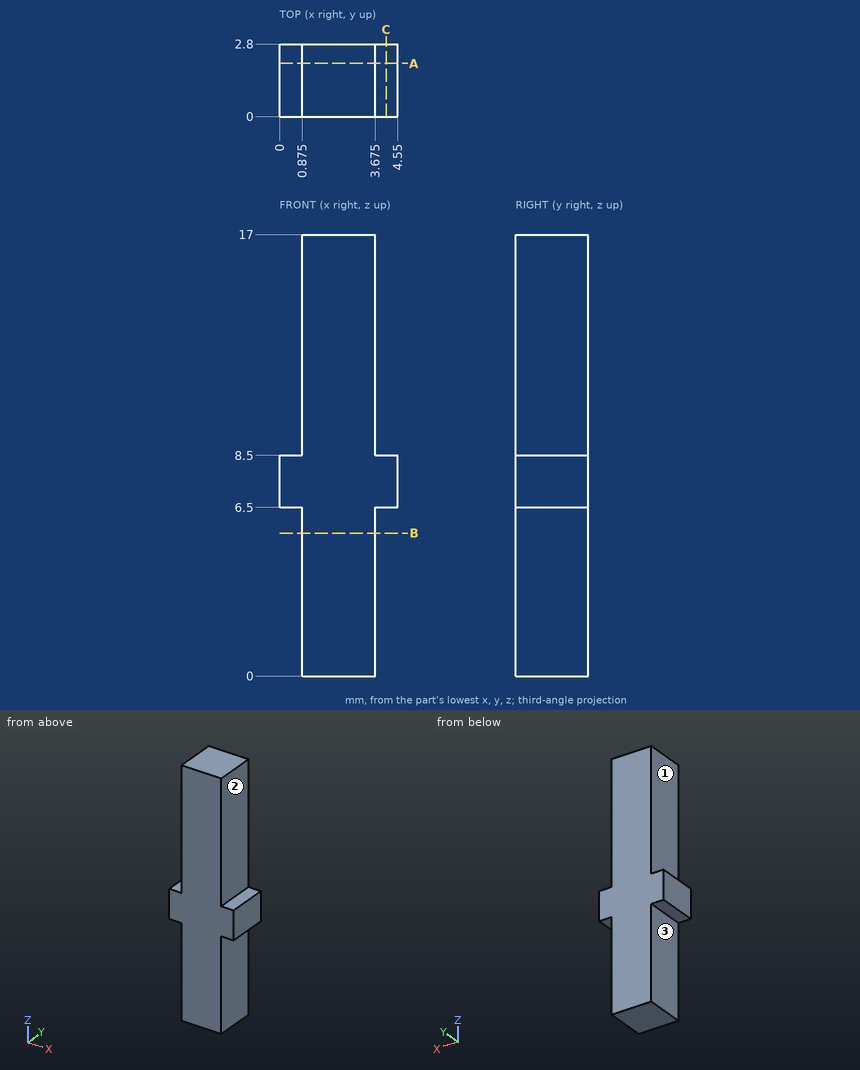
Study the drawing (mm; zero at the part's minimum x, y, z) and answer. A direction names the side the tool comes from. Give positions to 0.01 mm unless a question says otherwise; leave off trailing zeros. Order: outer loops, then holes, each group sorted by start corner. A loop starts at its lowest first (then second) coordinate and runs counter-clockwise, first axis right, second up. Notation, with made-up numbers: (63, 69.5) - (104, 69.5) arc R30 cw to (104, 92.5) - close; hole circle Ø6 at (71.5, 80). An arc over 180 degrees is marked (long way). Use one line per item in the form item = value. Start each with the question number.
(1) A cutting plane is placed at C-C, the plane x = 4.1. Write down the section's boundary in (y, z).
(2) A cutting plane is placed at B-B, the plane z = 5.5. Write down the section's boundary in (x, y) (3 decimals).
(3) A cutting plane is placed at A-A, the plane y = 2.05. Write down the section's boundary in (x, z) (3 decimals).
(4) Flat-ended cylindrical pins translate along their axes: pin 1 Ø0.8 at (y, z) = (1.5, 12) entering from +X (3 decimals); pin 2 Ø1.4 at (y, z) = (1.5, 11.5) entering from -X (3 decimals); pin 3 Ø1 at (x, y) = (4, 1) entering from -Z. Find the tip coordinate at first contact, or state that the pin passes through.
(5) Consider line 1 (X direction, y = 2.5, z = 5.25) (3 decimals); line 2 (Z direction, x = 0.7, y = 1.5). Determine where each line is inside the solid, lowest interval first. Write a range as from..to.
(6) For the marked faces 1, 2 and 3, determine the directions among +Z, -Z, +X, -X, +Y, -Y from which every point of the face is accessible in a straight line to the end or side of a thin tool.
Ans:
q1.outline = (0, 6.5) - (2.8, 6.5) - (2.8, 8.5) - (0, 8.5) - close
q2.outline = (0.875, 0) - (3.675, 0) - (3.675, 2.8) - (0.875, 2.8) - close
q3.outline = (0, 6.5) - (0.875, 6.5) - (0.875, 0) - (3.675, 0) - (3.675, 6.5) - (4.55, 6.5) - (4.55, 8.5) - (3.675, 8.5) - (3.675, 17) - (0.875, 17) - (0.875, 8.5) - (0, 8.5) - close
q4.pin_1 = 3.675
q4.pin_2 = 0.875
q4.pin_3 = 0
q5.line_1 = 0.875..3.675
q5.line_2 = 6.5..8.5
q6.face_1 = +Z, -X, +Y, -Y
q6.face_2 = +Z, +X, +Y, -Y
q6.face_3 = -Z, -X, +Y, -Y
